Source: CAD feature listing. Evaluate the final solid. Frame: model axes, mm. Face numbers are marked on the shaded views. A direction names the side the tool comes from. Coordinates: 2 decimals unless noted, no trailing zeros. Order: outer loops, then holes, each group sorted by start corner. A loop starts at its lowest first (then second) coordinate and runs counter-clockwise, first axis right, second up. Notation, with made-up numbers: (-10, -3) -> (37, -3) arc R36 ccw to (37, 36) -> close; hole circle Ø8 at (-19, 80). An arc over 180 degrees is marked (long way). Write item = value, one per line. Start each with the question number.
Item 1: Ray query, line 1 along Y through (x, z) = (-2.5, -0.45) (3 decimals); line 2 along X through (y, z) = (-3.25, -1.9). Return the intervals inside material, ascending. Write a range as [from, to].
Item 2: Section query C-C (x = -3.5). Output: boundary loops of the cut face in (y, z) (3 decimals).
Item 3: Section query D-D (z = 0.25). Output: boundary loops of the cut face in (x, y) (3 decimals), then the cut area to 3 significant figures.
Item 4: Contact query for flat-ended pins moving along their axis: pin 1 (2 mm diameter, centred on y = -2.5, z = 1.5, fed in from -X); pin 2 (1.2 mm diameter, centred on x = -1.5, z = -0.5, fed in from +Y) (3 decimals); pin 3 (3 mm diameter, centred on x = -3.5, y = -2, fed in from +Z). Output: stop coordinate, or through.
Item 5: Section query B-B (z = 1.9). Output: boundary loops of the cut face in (x, y) (3 decimals), then the cut area to 3 significant figures.
Item 6: Section query A-A (y = 0.5). Output: boundary loops of the cut face in (x, z).
Item 7: Set-up query: the marked faces 1, 2, 3, 4 and 5. Return all of +Z, -Z, +X, -X, +Y, -Y with unobstructed straight access to the full face (end or side cutting, diameter ignored); none if empty.
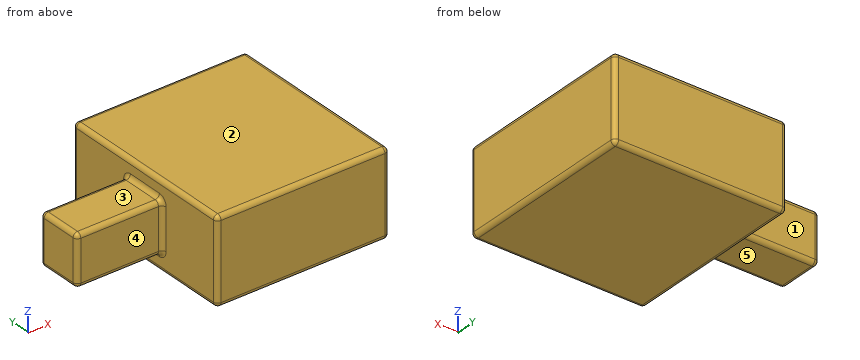
Autodesk Inventor part; units mm, degrees
ref_plane "YZ Plane" through (0, 0, 0) normal (1, 0, 0) x (0, 1, 0)
ref_plane "XZ Plane" through (0, 0, 0) normal (0, 1, 0) x (-1, 0, 0)
ref_plane "XY Plane" through (0, 0, 0) normal (0, 0, 1) x (1, 0, 0)
sketch "Sketch1" plane through (0, 0, 0) normal (1, 0, 0) x (0, 1, 0)
  line L0 (1.325, 1.45) -> (-1.325, 1.45)
  line L1 (-1.325, 1.45) -> (-1.325, -1.45)
  line L2 (-1.325, -1.45) -> (1.325, -1.45)
  line L3 (1.325, -1.45) -> (1.325, 1.45)
  point P0 (0, 0)
  dimension "d0" = 2.9
  dimension "d1" = 2.65
  dimension "d2" = 1.45
  dimension "d3" = 1.325
extrude "Extrusion1" add sketch "Sketch1" against normal blind 5
sketch "Sketch2" plane through (0, 0, 0) normal (1, 0, 0) x (0, 0, -1)
  line L0 (-2.45, 5.325) -> (2.45, 5.325)
  line L1 (2.45, 5.325) -> (2.45, -5.325)
  line L2 (2.45, -5.325) -> (-2.45, -5.325)
  line L3 (-2.45, -5.325) -> (-2.45, 5.325)
  line L4 (-1.45, 1.325) -> (-1.45, -1.325)
  line L5 (1.45, -1.325) -> (1.45, 1.325)
  line L6 (1.45, 1.325) -> (-1.45, 1.325)
  line L7 (-1.45, -1.325) -> (1.45, -1.325)
  point P0 (0, 0)
  dimension "d6" = 1
  dimension "d7" = 1
  dimension "d8" = 4
  dimension "d9" = 4
extrude "Extrusion2" add sketch "Sketch2" along normal blind 10 contours L0 L1 L2 L3 | L6 L5 L7 L4
fillet "Fillet1" radius 0.25 24 edges at (5, 5.325, 2.45) (5, 5.325, -2.45) (5, -5.325, -2.45) (5, -5.325, 2.45) (10, -5.325, 0) (10, 0, 2.45) (10, 0, -2.45) (10, 5.325, 0) (0, 5.325, 0) (0, -5.325, 0) (0, 0, 2.45) (0, 0, -2.45) (-2.5, 1.325, -1.45) (-2.5, 1.325, 1.45) (-2.5, -1.325, -1.45) (-2.5, -1.325, 1.45) (0, 1.325, 0) (0, 0, 1.45) (0, 0, -1.45) (0, -1.325, 0) (-5, 0, 1.45) (-5, 1.325, 0) (-5, 0, -1.45) (-5, -1.325, 0)
properties part number "dual_slider_paddlew"
Computed:
q1.line_1 = [-1.325, 1.325]
q1.line_2 = [0, 10]
q2.outline = (-1.325, -1.2) arc R0.25 ccw to (-1.075, -1.45) -> (1.075, -1.45) arc R0.25 ccw to (1.325, -1.2) -> (1.325, 1.2) arc R0.25 ccw to (1.075, 1.45) -> (-1.075, 1.45) arc R0.25 ccw to (-1.325, 1.2) -> close
q3.outline = (-5, -1.075) arc R0.25 ccw to (-4.75, -1.325) -> (-0.25, -1.325) arc R0.25 cw to (0, -1.575) -> (0, -5.075) arc R0.25 ccw to (0.25, -5.325) -> (9.75, -5.325) arc R0.25 ccw to (10, -5.075) -> (10, 5.075) arc R0.25 ccw to (9.75, 5.325) -> (0.25, 5.325) arc R0.25 ccw to (0, 5.075) -> (0, 1.575) arc R0.25 cw to (-0.25, 1.325) -> (-4.75, 1.325) arc R0.25 ccw to (-5, 1.075) -> close
q3.area = 120 mm^2
q4.pin_1 = 0
q4.pin_2 = 1.325
q4.pin_3 = 1.45
q5.outline = (0, -5.075) arc R0.25 ccw to (0.25, -5.325) -> (9.75, -5.325) arc R0.25 ccw to (10, -5.075) -> (10, 5.075) arc R0.25 ccw to (9.75, 5.325) -> (0.25, 5.325) arc R0.25 ccw to (0, 5.075) -> close
q5.area = 106 mm^2
q6.outline = (-5, -1.2) arc R0.25 ccw to (-4.75, -1.45) -> (-0.25, -1.45) arc R0.25 cw to (0, -1.7) -> (0, -2.2) arc R0.25 ccw to (0.25, -2.45) -> (9.75, -2.45) arc R0.25 ccw to (10, -2.2) -> (10, 2.2) arc R0.25 ccw to (9.75, 2.45) -> (0.25, 2.45) arc R0.25 ccw to (0, 2.2) -> (0, 1.7) arc R0.25 cw to (-0.25, 1.45) -> (-4.75, 1.45) arc R0.25 ccw to (-5, 1.2) -> close
q7.face_1 = +Z, -Z, -X, +Y
q7.face_2 = +Z, +X, -X, +Y, -Y
q7.face_3 = +Z, -X, +Y, -Y
q7.face_4 = +Z, -Z, -X, -Y
q7.face_5 = -Z, -X, +Y, -Y
